from build123d import *

# Parameters (mm, degrees)
SKETCH_1_R               = 20
EXTRUDE_1_DEPTH          = 15
SKETCH_2_R               = 2.5
CUT_EXTRUDE_1_DEPTH      = 10
MIRROR_2_COPY_1_SKETCH_R = 2.5
MIRROR_2_COPY_1_DEPTH    = 10
SKETCH_3_R               = 2.5
CUT_EXTRUDE_2_DEPTH      = 10
MIRROR_4_COPY_1_SKETCH_R = 2.5
MIRROR_4_COPY_1_DEPTH    = 10
SKETCH_4_R               = 1.5
CUT_EXTRUDE_3_DEPTH      = 87.365727496
PATTERN_CIRCULAR_1_COUNT = 6


with BuildPart() as part:
    # 草图1 → 凸台-拉伸1 (new body)
    with BuildSketch(Plane(origin=(0, 0, 0), x_dir=(1, 0, 0), z_dir=(0, 1, 0))):
        with BuildLine():
            Line((46.623322285, 16.328680875), (65.781966365, 25.910071498))
            ThreePointArc((65.781966365, 25.910071498), (68.576327064, 34.295567803), (60.190830759, 37.089928502))
            Line((60.190830759, 37.089928502), (41.03218668, 27.50853788))
            ThreePointArc((41.03218668, 27.50853788), (0, 49.4), (-41.03218668, 27.50853788))
            Line((-41.03218668, 27.50853788), (-60.190830759, 37.089928502))
            ThreePointArc((-60.190830759, 37.089928502), (-68.576327064, 34.295567803), (-65.781966365, 25.910071498))
            Line((-65.781966365, 25.910071498), (-46.623322285, 16.328680875))
            ThreePointArc((-46.623322285, 16.328680875), (-49.4, 0), (-46.623322285, -16.328680875))
            Line((-46.623322285, -16.328680875), (-65.781966365, -25.910071498))
            ThreePointArc((-65.781966365, -25.910071498), (-68.576327064, -34.295567803), (-60.190830759, -37.089928502))
            Line((-60.190830759, -37.089928502), (-41.03218668, -27.50853788))
            ThreePointArc((-41.03218668, -27.50853788), (0, -49.4), (41.03218668, -27.50853788))
            Line((41.03218668, -27.50853788), (60.190830759, -37.089928502))
            ThreePointArc((60.190830759, -37.089928502), (68.576327064, -34.295567803), (65.781966365, -25.910071498))
            Line((65.781966365, -25.910071498), (46.623322285, -16.328680875))
            ThreePointArc((46.623322285, -16.328680875), (49.4, 0), (46.623322285, 16.328680875))
        make_face()
        with Locations(Location((0, 0, 0), (0, 0, 270))):
            Circle(SKETCH_1_R, mode=Mode.SUBTRACT)
    extrude(amount=EXTRUDE_1_DEPTH)

    # 草图2 → 切除-拉伸1 (cut)
    with BuildSketch(Plane(origin=(0, 15, 0), x_dir=(1, 0, 0), z_dir=(0, 1, 0))):
        with Locations(Location((-62.986398562, 31.5, 0), (0, 0, 270))):
            Circle(SKETCH_2_R)
    cut_extrude_1 = extrude(amount=-CUT_EXTRUDE_1_DEPTH, mode=Mode.SUBTRACT)

    # 镜向1: 切除-拉伸1 across plane
    add(cut_extrude_1.mirror(Plane.XY), mode=Mode.SUBTRACT)

    # 镜向2: 切除-拉伸1 across plane
    add(cut_extrude_1.mirror(Plane(origin=(0, 0, 0), x_dir=(0, 0, 1), z_dir=(1, 0, 0))), mode=Mode.SUBTRACT)

    # 镜向2 copy 1 sketch → 镜向2 copy 1 (cut)
    with BuildSketch(Plane(origin=(0, 15, 0), x_dir=(-1, 0, 0), z_dir=(0, 1, 0))):
        with Locations(Location((-62.986398562, 31.5, 0), (0, 0, 270))):
            Circle(MIRROR_2_COPY_1_SKETCH_R)
    extrude(amount=-MIRROR_2_COPY_1_DEPTH, mode=Mode.SUBTRACT)

    # 草图3 → 切除-拉伸2 (cut)
    with BuildSketch(Plane.XZ):
        with Locations(Location((-54.042512958, 27.027091516, 0), (0, 0, 270))):
            Circle(SKETCH_3_R)
    cut_extrude_2 = extrude(amount=-CUT_EXTRUDE_2_DEPTH, mode=Mode.SUBTRACT)

    # 镜向3: 切除-拉伸2 across plane
    add(cut_extrude_2.mirror(Plane(origin=(0, 0, 0), x_dir=(0, 0, 1), z_dir=(1, 0, 0))), mode=Mode.SUBTRACT)

    # 镜向4: 切除-拉伸2 across plane
    add(cut_extrude_2.mirror(Plane.XY), mode=Mode.SUBTRACT)

    # 镜向4 copy 1 sketch → 镜向4 copy 1 (cut)
    with BuildSketch(Plane(origin=(0, 0, 0), x_dir=(-1, 0, 0), z_dir=(0, -1, 0))):
        with Locations(Location((-54.042512958, 27.027091516, 0), (0, 0, 270))):
            Circle(MIRROR_4_COPY_1_SKETCH_R)
    extrude(amount=-MIRROR_4_COPY_1_DEPTH, mode=Mode.SUBTRACT)

    # 草图4 → 切除-拉伸3 (cut, through all)
    with BuildSketch(Plane.XZ):
        with Locations(Location((0, -43.5, 0), (0, 0, 270))):
            Circle(SKETCH_4_R)
    cut_extrude_3 = extrude(amount=-CUT_EXTRUDE_3_DEPTH, mode=Mode.SUBTRACT)

    # 阵列(圆周)1: 切除-拉伸3 ×6 about axis
    pattern_circular_1_axis = Axis((0, 0, 0), (0, 1, 0))
    for i in range(1, PATTERN_CIRCULAR_1_COUNT):
        add(cut_extrude_3.rotate(pattern_circular_1_axis, i * 360 / PATTERN_CIRCULAR_1_COUNT), mode=Mode.SUBTRACT)


solid = part.part
Input: part model. Units: mm. Frame: model coordinates. A direction names the side the tool comes from. Give positions to 0.01 mm unless a question says otherwise; leave off trailing zeros. Write each loop counter-clockwise with the first axis right and the second up, starting at its lowest first coordinate (ties: lowest second). Pieces come first, ordered by that corner, then holes. Notation, with made-up numbers: (80.5, 61) -> (121.5, 61) arc R21 cw to (121.5, 75) -> close; hole circle Ø8 at (-38, 17.25). An arc over 180 degrees is marked (long way). Use one line per item in the form item = value. Start each with the question number.
1) Draft query along Z for faces 1 (the cylindrical face through (-68.636, 7.395, 34.172)), 2 (the flat face through (-50.477, 7.395, -32.232)), 3 (the flat face through (50.477, 7.395, 32.232)), 4 (the cylindrical face through (-68.514, 7.395, -34.418)). Return one class per face: pulls with the +Z half, pulls with the -Z half, needs draft (parallel to the pull), parting line crosses it, or undercut.
2) Section query B-B on x = 0. Return the cut outline in (y, z).
3) Section query A-A on z = 0. Return the cut outline in (x, y).
4) Section query D-D on x = -18. Return the cut outline in (y, z), then the cut area to 3 significant figures.
5) Set-up query: faces 5 (the flat face through (56.34, 7.4, 21.19)), 6 (the flat face through (-63, 5, -32)), 7 (the flat face through (54, 10, -27)), 8 (the flat face through (-50.75, 7.4, 32.37)). Return all of +Z, -Z, +X, -X, +Y, -Y with unobstructed straight access to the full face (end or side cutting, diameter ignored); none if empty.
6) Ray query, probe 1 along Z at (x, y) = (54, 1); probe 2 along X at (y, z) = (6.25, 0); probe 3 along X at (y, z) = (5, -21.75). Return the intervals inside material, ascending. Write a range as from..to.
7) Section query C-C on y = 8. Count the separate pieces of the cut face and the enclosed holes in it, then the cut area to 3 significant figures.
8) Pin query (flat end, axial travel): pin 1 (1.5 mm diameter, centred on x = 55.5, z = -27.5, fed in from -Y); pin 2 (2 mm diameter, centred on x = 30, z = 17.5, fed in from -Y); pin 3 (4 mm diameter, centred on y = 10, z = -25.5, fed in from +X); pin 4 (2 mm diameter, centred on x = 21, y = 4.5, fed in from -Z). Return the tip coordinate at first contact, or that it passes through.
Outcome:
q1.face_1 = undercut
q1.face_2 = pulls with the -Z half
q1.face_3 = pulls with the +Z half
q1.face_4 = undercut
q2.outline = (0, -49.4) -> (15, -49.4) -> (15, -45) -> (0, -45) -> close; (0, -42) -> (15, -42) -> (15, -20) -> (0, -20) -> close; (0, 20) -> (15, 20) -> (15, 42) -> (0, 42) -> close; (0, 45) -> (15, 45) -> (15, 49.4) -> (0, 49.4) -> close
q3.outline = (-49.4, 0) -> (-20, 0) -> (-20, 15) -> (-49.4, 15) -> close; (20, 0) -> (49.4, 0) -> (49.4, 15) -> (20, 15) -> close
q4.outline = (0, -46) -> (15, -46) -> (15, -8.72) -> (0, -8.72) -> close; (0, 8.72) -> (15, 8.72) -> (15, 46) -> (0, 46) -> close
q4.area = 1,120 mm^2
q5.face_5 = +X, +Y, -Y
q5.face_6 = +Y
q5.face_7 = -Y
q5.face_8 = +Z, +Y, -Y
q6.probe_1 = -33.99..-29.53, -24.53..-20.02, 20.02..24.53, 29.53..33.99
q6.probe_2 = -49.4..-20, 20..49.4
q6.probe_3 = -57.46..-39.17, -36.17..36.17, 39.17..57.46
q7.separate_pieces = 1
q7.enclosed_holes = 15
q7.area = 7,510 mm^2
q8.pin_1 = 10
q8.pin_2 = 0
q8.pin_3 = 67.79
q8.pin_4 = -45.17
